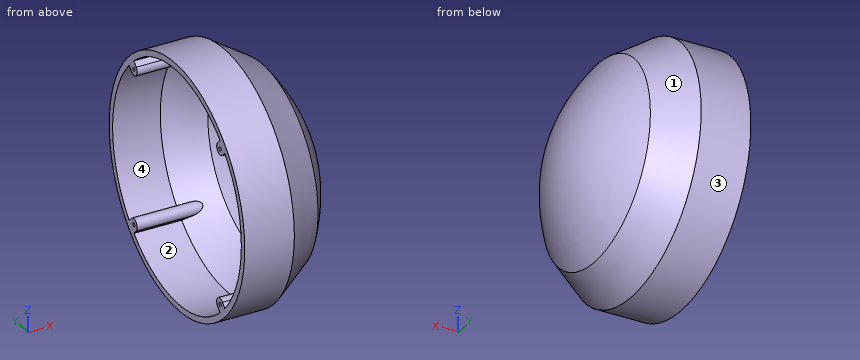
```python
from build123d import *

# Parameters (mm, degrees)
SURFACE_EXTRUDE3_1_DEPTH = 20
THICKEN6_T1              = 2.5
BOSS_EXTRUDE2_DEPTH      = 20
SKETCH6_R                = 0.75
CUT_EXTRUDE1_DEPTH       = 74.484692283
BOSS_EXTRUDE4_REACH      = 75.485
THICKEN8_T1              = 2.5
BODY_MOVE_COPY1_ANGLE    = 45


# Read off the part's stored shape, not the designer's step: Thicken7
with BuildPart() as body_1:
    # Surface-Extrude3: a surface, the sketch's curves swept straight by 20 mm
    with BuildLine(Plane(origin=(0, 0, 0), x_dir=(0, 0, -1), z_dir=(1, 0, 0)), mode=Mode.PRIVATE) as surface_extrude3_1_path:
        CenterArc((0, 0), 50, 0, 360)
    surface_extrude3_1 = Shell.extrude(surface_extrude3_1_path.wire(), (1 * SURFACE_EXTRUDE3_1_DEPTH, 0 * SURFACE_EXTRUDE3_1_DEPTH, 0 * SURFACE_EXTRUDE3_1_DEPTH))
    add(Solid.thicken(surface_extrude3_1, THICKEN6_T1))

    # Sketch5 → Boss-Extrude2 (add)
    with BuildSketch(Plane(origin=(0, 0, 0), x_dir=(0, 0, -1), z_dir=(1, 0, 0))):
        with BuildLine():
            Line((2.5, 45), (2.5, 47.5))
            Line((2.5, 47.5), (-2.5, 47.5))
            Line((-2.5, 47.5), (-2.5, 45))
            ThreePointArc((-2.5, 45), (0, 42.5), (2.5, 45))
        make_face()
        with BuildLine():
            Line((-45, -2.5), (-47.5, -2.5))
            Line((-47.5, -2.5), (-47.5, 2.5))
            Line((-47.5, 2.5), (-45, 2.5))
            ThreePointArc((-45, 2.5), (-42.5, 0), (-45, -2.5))
        make_face()
        with BuildLine():
            Line((47.5, 2.5), (45, 2.5))
            ThreePointArc((45, 2.5), (42.5, 0), (45, -2.5))
            Line((45, -2.5), (47.5, -2.5))
            Line((47.5, -2.5), (47.5, 2.5))
        make_face()
        with BuildLine():
            Line((-2.5, -47.5), (2.5, -47.5))
            Line((2.5, -47.5), (2.5, -45))
            ThreePointArc((2.5, -45), (0, -42.5), (-2.5, -45))
            Line((-2.5, -45), (-2.5, -47.5))
        make_face()
    extrude(amount=BOSS_EXTRUDE2_DEPTH)

    # Sketch6 → Cut-Extrude1 (cut, through all)
    with BuildSketch(Plane(origin=(0, 0, 0), x_dir=(0, 0, -1), z_dir=(1, 0, 0))):
        with Locations((0, 45)):
            Circle(SKETCH6_R)
        with Locations((45, 0)):
            Circle(SKETCH6_R)
        with Locations((0, -45)):
            Circle(SKETCH6_R)
        with Locations((-45, 0)):
            Circle(SKETCH6_R)
    extrude(amount=CUT_EXTRUDE1_DEPTH, mode=Mode.SUBTRACT)

    # Thicken7 outline → Thicken7 (revolve)
    with BuildSketch(Plane.YX):
        Polygon((40, 35), (37.919874264, 33.613249509), (47.5, 19.243060906), (47.5, 20), (50, 20), align=None)
    revolve(axis=Axis((0, 0, 0), (1, 0, 0)))

    # Sketch10 → Boss-Extrude4 (add, up to next)
    with BuildSketch(Plane(origin=(20, 0, 0), x_dir=(0, 0, -1), z_dir=(1, 0, 0)), mode=Mode.PRIVATE) as boss_extrude4_sk1:
        with BuildLine():
            Line((-45, 2.5), (-46.92883092, 2.5))
            ThreePointArc((-46.92883092, 2.5), (-46.995373937, 0), (-46.92883092, -2.5))
            Line((-46.92883092, -2.5), (-45, -2.5))
            ThreePointArc((-45, -2.5), (-42.5, 0), (-45, 2.5))
        make_face()
    boss_extrude4_tool1 = extrude(boss_extrude4_sk1.sketch, amount=BOSS_EXTRUDE4_REACH, mode=Mode.PRIVATE) - body_1.part
    # Sketch10 → Boss-Extrude4 (add, up to next)
    with BuildSketch(Plane(origin=(20, 0, 0), x_dir=(0, 0, -1), z_dir=(1, 0, 0)), mode=Mode.PRIVATE) as boss_extrude4_sk2:
        with BuildLine():
            Line((-2.5, -45), (-2.5, -46.92883092))
            ThreePointArc((-2.5, -46.92883092), (0, -46.995373937), (2.5, -46.92883092))
            Line((2.5, -46.92883092), (2.5, -45))
            ThreePointArc((2.5, -45), (0, -42.5), (-2.5, -45))
        make_face()
    boss_extrude4_tool2 = extrude(boss_extrude4_sk2.sketch, amount=BOSS_EXTRUDE4_REACH, mode=Mode.PRIVATE) - body_1.part
    # Sketch10 → Boss-Extrude4 (add, up to next)
    with BuildSketch(Plane(origin=(20, 0, 0), x_dir=(0, 0, -1), z_dir=(1, 0, 0)), mode=Mode.PRIVATE) as boss_extrude4_sk3:
        with BuildLine():
            Line((45, -2.5), (46.92883092, -2.5))
            ThreePointArc((46.92883092, -2.5), (46.995373937, 0), (46.92883092, 2.5))
            Line((46.92883092, 2.5), (45, 2.5))
            ThreePointArc((45, 2.5), (42.5, 0), (45, -2.5))
        make_face()
    boss_extrude4_tool3 = extrude(boss_extrude4_sk3.sketch, amount=BOSS_EXTRUDE4_REACH, mode=Mode.PRIVATE) - body_1.part
    # Sketch10 → Boss-Extrude4 (add, up to next)
    with BuildSketch(Plane(origin=(20, 0, 0), x_dir=(0, 0, -1), z_dir=(1, 0, 0)), mode=Mode.PRIVATE) as boss_extrude4_sk4:
        with BuildLine():
            Line((2.5, 45), (2.5, 46.92883092))
            ThreePointArc((2.5, 46.92883092), (0, 46.995373937), (-2.5, 46.92883092))
            Line((-2.5, 46.92883092), (-2.5, 45))
            ThreePointArc((-2.5, 45), (0, 42.5), (2.5, 45))
        make_face()
    boss_extrude4_tool4 = extrude(boss_extrude4_sk4.sketch, amount=BOSS_EXTRUDE4_REACH, mode=Mode.PRIVATE) - body_1.part
    add(boss_extrude4_tool1.solids().sort_by_distance((20, 0, 44.965357))[0])
    add(boss_extrude4_tool2.solids().sort_by_distance((20, -44.965357, 0))[0])
    add(boss_extrude4_tool3.solids().sort_by_distance((20, 0, -44.965357))[0])
    add(boss_extrude4_tool4.solids().sort_by_distance((20, 44.965357, 0))[0])

    # Surface-Revolve3: a surface, the sketch's curves turned about an axis
    with BuildLine(Plane.XY, mode=Mode.PRIVATE) as surface_revolve3_2_path:
        add(Edge.make_bspline(
            [(35, 40), (50, 20), (50, 0)],
            knots=[0, 0, 0, 0.5, 0.5, 0.5], degree=2))
    surface_revolve3_2 = Shell.revolve(surface_revolve3_2_path.wire(), 360, Axis((50, 0, 0), (-1, 0, 0)))
    add(Solid.thicken(surface_revolve3_2, THICKEN8_T1))


with BuildPart() as body_1_1:
    # Body-Move/Copy1: moved
    add(body_1.part.rotate(Axis((0, 0, 0), (1, 0, 0)), BODY_MOVE_COPY1_ANGLE))


solid = body_1_1.part
```
Here's how the part is built. I have some questions about the finished solid (model axes, mm). Face numbers are marked on the shaded views. A direction names the side the tool comes from. Coordinates: 2 decimals unless noted, no trailing zeros. Order: outer loops, then holes, each group sorted by start corner. A loop starts at its lowest first (then second) coordinate and runs counter-clockwise, first axis right, second up. Notation, with made-up numbers: (67, 59) -> (81, 59) arc R21 ccw to (81, 91) -> close; hole circle Ø8 at (10.5, 84.5). An arc over 180 degrees is marked (long way). Return JSON: item names as keys, results as strings.
1) On a 3-axis mill with a long thin cutter (end or side, diameter ignored), from which of +Z, -Z, +X, -X, +Y, -Y can I reach the whole of each face in a straight line? I mean the marked faces 1 and 2. Say none if no direction works.
Conclusion:
{"face 1": "+X", "face 2": "-X"}
2) If I drill on probe 1 along Y at (x, z) = (9, -1.5); probe 2 along Z at (x, y) = (17, -1); probe 3 along Z at (x, y) = (6.5, -5), over which ranges is the centre line in solid material (lowest first)?
Conclusion:
{"probe 1": "y = -49.98 to -47.48, 47.48 to 49.98", "probe 2": "z = -49.99 to -47.49, 47.49 to 49.99", "probe 3": "z = -49.75 to -47.24, 47.24 to 49.75"}
3) Thinking about a two-plate mould opening in Y: for the marked faces 3 and 4, which applies, +Y half, -Y half, draft (parallel to the pull), parting line (faces both ways), or undercut?
Conclusion:
{"face 3": "parting line", "face 4": "undercut"}
4) I'm going to push flat-ended pins straight in: P1, Ø1.2, axis at y = 31.82, z = 31.82, coming from the +X side; P2, Ø1.2, axis at y = 31.5, z = 32, coming from the -X side; P3, Ø6, axis at y = 11, z = 32, coming from the -X side; P4, Ø1.7, axis at y = 31.82, z = -31.82, coming from the +X side. Where does each tip first touch, or does it pass through?
Conclusion:
{"P1": "stops at x = 28.4", "P2": "stops at x = 0", "P3": "stops at x = 34.22", "P4": "stops at x = 28.77"}
5) If we section it at A-A on x = 30: List the corners of the cut face in (y, z) for me, plus the area to 3 significant figures.
Conclusion:
{"outline": "circle Ø86.67 at (0, 0); hole circle Ø80.66 at (0, 0)", "area": "790 mm²"}
